Autodesk Inventor part; units mm, degrees
ref_plane "YZ Plane" through (0, 0, 0) normal (1, 0, 0) x (0, 1, 0)
ref_plane "XZ Plane" through (0, 0, 0) normal (0, 1, 0) x (-1, 0, 0)
ref_plane "XY Plane" through (0, 0, 0) normal (0, 0, 1) x (1, 0, 0)
sketch "Esboço1" plane through (0, 0, 0) normal (0, 1, 0) x (-1, 0, 0)
  line L0 (-17.7, -33) -> (17.7, -33)
  line L1 (17.7, -33) -> (17.7, 33)
  line L2 (17.7, 33) -> (-17.7, 33)
  line L3 (-17.7, 33) -> (-17.7, -33)
  line L4 (-17.7, -33) -> (17.7, 33) construction
  line L5 (17.7, -33) -> (-17.7, 33) construction
  circle A0 centre (15.55, 30.85) radius 1.35
  circle A1 centre (-15.55, 30.85) radius 1.35
  circle A2 centre (15.55, -30.85) radius 1.35
  circle A3 centre (-15.55, -30.85) radius 1.35
  point P0 (0, 0)
  dimension "d0" = 35.4
  dimension "d1" = 66
  dimension "d2" = 2.7
  dimension "d4" = 0.8
  dimension "d5" = 0.8
  dimension "d6" = 2.7
  dimension "d8" = 0.8
  dimension "d9" = 0.8
extrude "Extrusão1" add sketch "Esboço1" along normal blind 1.5
sketch "Esboço2" plane through (0, 1.5, 0) normal (0, 1, 0) x (1, 0, 0)
  line L0 (5, 24.7918) -> (-5, 24.7918)
  line L1 (-5, 24.7918) -> (-5, 32.6918)
  line L2 (-5, 32.6918) -> (5, 32.6918)
  line L3 (5, 32.6918) -> (5, 24.7918)
  line L4 (5, 24.7918) -> (-5, 32.6918) construction
  line L5 (-5, 24.7918) -> (5, 32.6918) construction
  line L6 (-26.0305, 0) -> (25.0606, 0)
  line L7 (5, -24.7918) -> (-5, -24.7918)
  line L8 (-5, -24.7918) -> (-5, -32.6918)
  line L9 (-5, -32.6918) -> (5, -32.6918)
  line L10 (5, -32.6918) -> (5, -24.7918)
  line L11 (16.2337, -11.3) -> (2.0337, -11.3)
  line L12 (2.0337, -11.3) -> (2.0337, 11.3)
  line L13 (2.0337, 11.3) -> (16.2337, 11.3)
  line L14 (16.2337, 11.3) -> (16.2337, -11.3)
  line L15 (16.2337, -11.3) -> (2.0337, 11.3) construction
  line L16 (2.0337, -11.3) -> (16.2337, 11.3) construction
  line L17 (-7.8666, -23.8534) -> (-2.8666, -23.8534)
  line L18 (-2.8666, -23.8534) -> (-2.8666, -18.8534)
  line L19 (-2.8666, -18.8534) -> (-7.8666, -18.8534)
  line L20 (-7.8666, -18.8534) -> (-7.8666, -23.8534)
  line L21 (-7.8666, 23.8534) -> (-2.8666, 23.8534)
  line L22 (-2.8666, 23.8534) -> (-2.8666, 18.8534)
  line L23 (-2.8666, 18.8534) -> (-7.8666, 18.8534)
  line L24 (-7.8666, 18.8534) -> (-7.8666, 23.8534)
  line L25 (11.4703, 16.4532) -> (15.4703, 16.4532)
  line L26 (15.4703, 16.4532) -> (15.4703, 20.4532)
  line L27 (15.4703, 20.4532) -> (11.4703, 20.4532)
  line L28 (11.4703, 20.4532) -> (11.4703, 16.4532)
  line L29 (-16.3029, 1.3386) -> (-12.8029, 1.3386)
  line L30 (-12.8029, 1.3386) -> (-12.8029, 9.3386)
  line L31 (-12.8029, 9.3386) -> (-16.3029, 9.3386)
  line L32 (-16.3029, 9.3386) -> (-16.3029, 1.3386)
  line L33 (-9.8893, 1.3386) -> (0, 1.3386)
  line L34 (0, 1.3386) -> (0, 11.3)
  line L35 (0, 11.3) -> (-9.8893, 11.3)
  line L36 (-9.8893, 11.3) -> (-9.8893, 1.3386)
  line L37 (-16.3029, -11.3) -> (-10.3029, -11.3)
  line L38 (-10.3029, -11.3) -> (-10.3029, -5.3)
  line L39 (-10.3029, -5.3) -> (-16.3029, -5.3)
  line L40 (-16.3029, -5.3) -> (-16.3029, -11.3)
  circle A0 centre (-15.55, -30.85) radius 1.35
  circle A1 centre (-15.55, -30.85) radius 1.65
  circle A2 centre (15.55, -30.85) radius 1.35
  circle A3 centre (15.55, -30.85) radius 1.65
  circle A4 centre (-15.55, 30.85) radius 1.65
  circle A5 centre (15.55, 30.85) radius 1.65
  point P0 (0, 0)
  point P1 (0, 28.7418)
  point P2 (0, -28.7418)
  point P3 (9.1337, 0)
  dimension "d12" = 10
  dimension "d13" = 7.9
  dimension "d14" = 14.2
  dimension "d15" = 22.6
  dimension "d16" = 5
  dimension "d17" = 5
  dimension "d18" = 4
  dimension "d19" = 4
  dimension "d20" = 3.5
  dimension "d21" = 8
  dimension "d22" = 6
  dimension "d23" = 6
  dimension "d42" = 3.3
  dimension "d43" = 3.3
extrude "Extrusão2" add sketch "Esboço2" along normal blind 10 contours L0 L1 L2 L3 | L10 L9 L8 L7 | L32 L31 L30 L29
chamfer "Chanfro1" distance 2 angle 45 4 edges at (0, 11.5, -24.7918) (0, 11.5, -32.6918) (0, 11.5, 32.6918) (0, 11.5, 24.7918)
extrude "Extrusão3" add sketch "Esboço2" along normal blind 7.5 contours L12 L13 L14 L6 | L6 L14 L11 L12 | L36 L35 L34 L33
extrude "Extrusão4" add sketch "Esboço2" along normal blind 3 contours L28 L27 L26 L25 | L40 L39 L38 L37
extrude "Extrusão5" add sketch "Esboço2" along normal blind 1.5 contours L20 L19 L18 L17 | L21 L22 L23 L24
sketch "Esboço3" plane through (0, 3, 0) normal (0, 1, 0) x (1, 0, 0)
  line L0 (-7.8666, -18.8534) -> (-7.8666, -23.8534)
  line L1 (-7.8666, -23.8534) -> (-2.8666, -23.8534)
  line L2 (-2.8666, -18.8534) -> (-7.8666, -18.8534)
  line L3 (-2.8666, -23.8534) -> (-2.8666, -18.8534)
  circle A0 centre (-5.3666, -21.3534) radius 2.5
  point P0 (0, 0)
sketch "Esboço4" plane through (0, 3, 0) normal (0, 1, 0) x (1, 0, 0)
  line L0 (-7.8666, 23.8534) -> (-7.8666, 18.8534)
  line L1 (-7.8666, 18.8534) -> (-2.8666, 18.8534)
  line L2 (-2.8666, 23.8534) -> (-7.8666, 23.8534)
  line L3 (-2.8666, 18.8534) -> (-2.8666, 23.8534)
  circle A0 centre (-5.3666, 21.3534) radius 2.5
  point P0 (0, 0)
sketch "Esboço7" plane through (0, 4.5, 0) normal (0, 1, 0) x (1, 0, 0)
  line L0 (11.4703, 20.4532) -> (11.4703, 16.4532)
  line L1 (11.4703, 16.4532) -> (15.4703, 16.4532)
  line L2 (15.4703, 20.4532) -> (11.4703, 20.4532)
  line L3 (15.4703, 16.4532) -> (15.4703, 20.4532)
  circle A0 centre (13.4703, 18.4532) radius 1.5205
  point P0 (0, 0)
extrude "Extrusão6" add sketch "Esboço3" along normal blind 11 contours A0
extrude "Extrusão7" add sketch "Esboço4" along normal blind 11 contours A0
extrude "Extrusão8" add sketch "Esboço7" along normal blind 1 contours A0
fillet "Arredondamento1" radius 1 2 edges at (-7.8666, 14, 21.3534) (-7.8666, 14, -21.3534)
extrude "Extrusão9" cut sketch "Esboço2" against normal blind 0.1 contours A1 | A3 | A4 | A5
properties part number "STEP_DOWN_LM2596"
Geometry: final body of the model. Coordinates: model frame, mm. A direction names the side the tool comes from. Round coordinates to 2 decimals unless told otherwise and drop trailing zeros. Write each loop counter-clockwise with the first axis right and the second up, starting at its lowest first coordinate (ties: lowest second). Pieces come first, ordered by that corner, then holes. Notation, with made-up numbers: (35, -30) -> (81, -30) arc R24 cw to (81, -5) -> close; hole circle Ø9 at (19.25, 84). An arc over 180 degrees is marked (long way). Use CSV: the item, a comma, the result in double quotes. Start each with the question number.
Q1. Pull-direction query (X, two-part tool) for faces 1 (the face through (11.47, 3, -18)), 2 (the face through (-7.4, 3, 23.2)), 3 (the face through (-7.867, 2, 21)); classes: pulls with the +X half, pulls with the -X half, needs draft (parallel to the pull), parting line crosses it, or undercut.
Q2. Reachability of faces 4 (the face through (-16.303, 3, 8)), 5 (the face through (0, 5, -24.792)), 6 (the face through (-3.4, 3, 23.3)), 7 (the face through (-13, 3, 11.3)), 8 (the face through (-13, 4.5, 8)) from +Z, -Z, +X, -X, +Y, -Y: full face, straight path, thin tool, end or side. Return the list, or none.
Q3. First-contact query: pin 1 Ø3.5 at (x, z) = (14, -18.5) entering from +Y; pin 2 Ø3 at (y, z) = (7.5, -23.5) entering from +X; pin 3 Ø12 at (x, z) = (1.5, -2.5) entering from +Y. Flat tips, straight axial feed; report the tip coordinate or a pass-through.
Q4. Section A-A (z = 7.5). Return loops of the section in (x, y).
Q5. Section D-D (x = 6). Return loops of the section in (y, z), plus the area to 4 significant figures.
Q6. Section C-C (y = 10.5). Return loops of the section in (x, z).
Q7. Section B-B (x = -15.55). Return loops of the section in (y, z).
Q8. Line query: L1, parallel to Z at x = 3.5, y = 8.5; L2, parallel to X at y = 1.45, z = 30.85; L3, parallel to Z at x = -5.5, y = 2.5. Output: solid intervals per line, ascending.
Result sheet:
1,face 1,"undercut"
1,face 2,"needs draft"
1,face 3,"pulls with the -X half"
2,face 4,"+Z, -Z, -X, +Y"
2,face 5,"+X, -X, +Y"
2,face 6,"+X, +Y"
2,face 7,"+Z, +X, -X, +Y"
2,face 8,"+Z, -X, +Y"
3,pin 1,"y = 5.5"
3,pin 2,"x = 5"
3,pin 3,"y = 9"
4,outline,"(-17.7, 0) -> (17.7, 0) -> (17.7, 1.5) -> (16.23, 1.5) -> (16.23, 9) -> (2.03, 9) -> (2.03, 1.5) -> (-10.3, 1.5) -> (-10.3, 4.5) -> (-16.3, 4.5) -> (-16.3, 1.5) -> (-17.7, 1.5) -> close"
5,outline,"(0, -33) -> (1.5, -33) -> (1.5, -11.3) -> (9, -11.3) -> (9, 11.3) -> (1.5, 11.3) -> (1.5, 33) -> (0, 33) -> close"
5,area,"268.5 mm²"
6,outline,"(-16.3, -9.34) -> (-12.8, -9.34) -> (-12.8, -1.34) -> (-16.3, -1.34) -> close; circle Ø5 at (-5.37, -21.35); circle Ø5 at (-5.37, 21.35); (-5, -31.69) -> (5, -31.69) -> (5, -25.79) -> (-5, -25.79) -> close; (-5, 25.79) -> (5, 25.79) -> (5, 31.69) -> (-5, 31.69) -> close"
7,outline,"(0, -33) -> (1.5, -33) -> (1.5, -32.5) -> (1.4, -32.5) -> (1.4, -32.2) -> (0, -32.2) -> close; (0, -29.5) -> (1.4, -29.5) -> (1.4, -29.2) -> (1.5, -29.2) -> (1.5, -9.34) -> (11.5, -9.34) -> (11.5, -1.34) -> (1.5, -1.34) -> (1.5, 5.3) -> (4.5, 5.3) -> (4.5, 11.3) -> (1.5, 11.3) -> (1.5, 29.2) -> (1.4, 29.2) -> (1.4, 29.5) -> (0, 29.5) -> close; (0, 32.2) -> (1.4, 32.2) -> (1.4, 32.5) -> (1.5, 32.5) -> (1.5, 33) -> (0, 33) -> close"
8,L1,"-32.69 to -24.79, -11.3 to 11.3, 24.79 to 32.69"
8,L2,"-17.7 to -17.2, -13.9 to 13.9, 17.2 to 17.7"
8,L3,"-23.85 to -18.85, -11.3 to -1.34, 18.85 to 23.85"
